Read the model definition and answer for the solid it produces. Units are mm, in the model's axes. A direction names the side the tool comes from. Coordinates: 2 decimals unless noted, no trailing zeros. Loops run counter-clockwise (first coordinate to the right, second up) from the corner with the lowest first, then second, coordinate; pieces in that order, holes last. Notation, with made-up numbers: M 77,-2.75 L 102,-2.75 A15 ccw 102,18.25 Z; hole C 18.25,80.25 d3. An arc over 180 degrees is marked long. One line per item, written item: value. Start each with the question number.
1. The part is cut by section D-D (z = 32). Write down the section's boundary in (x, y).
2. The part is cut by section B-B (y = 2). Write down the section's boundary in (x, z).
3. For faces 1 (the face through (-25, 50.8, 28)), 2 (the face through (-38.655, 33.572, 45.501)), 3 (the face through (36.83, 0, -13)), determine the directions among +Z, -Z, +X, -X, +Y, -Y from which every point of the face is accessible in a straight line to the end or side of a thin tool.
4. The part is cut by section C-C (x = 13.5). Write down the section's boundary in (y, z), then the cut area to 3 significant figures.
5. The part is cut by section A-A (z = 6). Write down the section's boundary in (x, y), then the cut area to 3 significant figures.
6. Determine the mould class of faces 4 (the face through (38.13, -0.71, -11.87)), 5 (the face through (-42.385, -26.625, 54.213)), 6 (the face through (-25, -50.8, 28)), 7 (the face through (-11.24, -0.71, -15.74)) for opening direction Z: +Z half, -Z half, draft (parallel to the pull), parting line (faces both ways), or undercut.
7. Consider probe 1 along Y at (x, z) = (-9.5, 4.5); probe 2 along Y at (x, z) = (-76.5, 23.5); probe 3 along Z at (x, y) = (-40.5, -30.5). Determine where each line is inside the solid, lowest interval first.
8. Flat-ended cylindrical pins translate along their axes: pin 1 (10 mm diameter, centred on x = -50, y = -8.5, fed in from -Z); pin 2 (3.5 mm diameter, centred on y = -3, z = -13.5, fed in from -X); pin 3 (5 mm diameter, centred on x = -2.5, y = 3.5, fed in from +Z). Find the tip coordinate at first contact, or state that the pin passes through.
```python
from build123d import *

# Parameters (mm, degrees)
F1_DEPTH      = 50.8
F3_DEPTH      = 110.998
F3_DEPTH_BACK = 36.83


with BuildPart() as f1:
    # F0 (on Front) → F1 (new body, symmetric)
    with BuildSketch(Plane.XZ):
        with BuildLine():
            ThreePointArc((-67.1143651523, 11.3118788967), (-27.3595519648, 13.4827854023), (-8.0827849332, 48.3190346183))
            ThreePointArc((-8.0827849332, 48.3190346183), (-9.7368789489, 59.8638451946), (-14.5660720417, 70.4797564755))
            ThreePointArc((-14.5660720417, 70.4797564755), (-79.9405579391, 75.6216888269), (-67.1143651523, 11.3118788967))
        make_face()
        with BuildLine():
            ThreePointArc((-14.5660720417, 70.4797564755), (-9.7368789489, 59.8638451946), (-8.0827849332, 48.3190346183))
            ThreePointArc((-8.0827849332, 48.3190346183), (-27.3595519648, 13.4827854023), (-67.1143651523, 11.3118788967))
            Line((-67.1143651523, 11.3118788967), (25.3778976938, -33.4652555138))
            ThreePointArc((25.3778976938, -33.4652555138), (21.608634566, -14.5663819856), (40.8203868988, -16.0774536137))
            Line((40.8203868988, -16.0774536137), (-14.5660720417, 70.4797564755))
        make_face()
        with BuildLine():
            ThreePointArc((42.7256455715, -22.589876526), (42.2395531131, -19.1971761709), (40.8203868988, -16.0774536137))
            ThreePointArc((40.8203868988, -16.0774536137), (21.608634566, -14.5663819856), (25.3778976938, -33.4652555138))
            ThreePointArc((25.3778976938, -33.4652555138), (37.0607371764, -32.8272861661), (42.7256455715, -22.589876526))
        make_face()
    extrude(amount=F1_DEPTH, both=True)

    # F2 (on Right) → F3 (cut, two sides)
    with BuildSketch(Plane.YZ) as f3_sk:
        Polygon((-13.2447925757, 66.9455137627), (-40.3845238139, 41.1189961655), (-37.1138849261, 3.7977295184), (-5.8957337036, -16.9146111783), (29.7620252487, -5.4212109251), (43.0083721541, 29.6231654646), (23.8685376165, 61.8293877944), align=None)
    extrude(amount=-F3_DEPTH, mode=Mode.SUBTRACT)
    extrude(f3_sk.sketch, amount=F3_DEPTH_BACK, mode=Mode.SUBTRACT)


solid = f1.part
```
Answer block:
1. outline: M -86.94,-50.8 L 10.06,-50.8 L 10.06,-39.59 L -86.94,-39.59 Z; M -86.94,41.6 L 10.06,41.6 L 10.06,50.8 L -86.94,50.8 Z
2. outline: M -86.85,64.84 L -10.96,64.84 L -14.57,70.48 A41.12 ccw Z; M -14.07,-14.37 L 25.38,-33.47 A12.08 ccw 40.82,-16.08 L 36.83,-9.84 L 36.83,-14.37 Z
3. face 1: +Z, -Z, +X, -X, +Y
3. face 2: +X, -X
3. face 3: +Z, -X
4. outline: M -50.8,-27.71 L 50.8,-27.71 L 50.8,26.62 L 41.87,26.62 L 29.76,-5.42 L -5.9,-16.91 L -37.11,3.8 L -39.11,26.62 L -50.8,26.62 Z
4. area: 2,920 mm2
5. outline: M -56.14,-50.8 L 26.69,-50.8 L 26.69,-37.31 L -56.14,-37.31 Z; M -56.14,34.08 L 26.69,34.08 L 26.69,50.8 L -56.14,50.8 Z
5. area: 2,500 mm2
6. face 4: +Z half
6. face 5: undercut
6. face 6: draft
6. face 7: -Z half
7. probe 1: y = -50.8 to -37.18, 33.51 to 50.8
7. probe 2: y = -50.8 to -38.84, 40.69 to 50.8
7. probe 3: z = -1.57 to -0.59, 50.53 to 88.5
8. pin 1: stops at z = 65.6
8. pin 2: stops at x = 36.83
8. pin 3: stops at z = -13.08
